from build123d import *

# Parameters (mm, degrees)
SKETCH_1_W      = 11.1
SKETCH_1_H      = 9.9
EXTRUDE_1_DEPTH = 5
SKETCH_1_3_W    = 7
SKETCH_1_3_H    = 9.9
EXTRUDE_2_DEPTH = 10
CHAMFER_1_SIZE  = 1


with BuildPart() as part:
    # 스케치1 → 보스-돌출1 (new body)
    with BuildSketch(Plane.XY):
        Rectangle(SKETCH_1_W, SKETCH_1_H)
    extrude(amount=EXTRUDE_1_DEPTH)

    # 스케치1<3> → 보스-돌출2 (add)
    with BuildSketch(Plane.XY):
        with Locations((-9.05, 0)):
            Rectangle(SKETCH_1_3_W, SKETCH_1_3_H)
        with Locations((9.05, 0)):
            Rectangle(SKETCH_1_3_W, SKETCH_1_3_H)
    extrude(amount=EXTRUDE_2_DEPTH)

    # 모따기1
    chamfer_1_edges = [part.edges().sort_by_distance(p)[0] for p in [
        (-12.55, 0, 0),
        (12.55, 0, 0),
    ]]
    chamfer(chamfer_1_edges, length=CHAMFER_1_SIZE)


solid = part.part
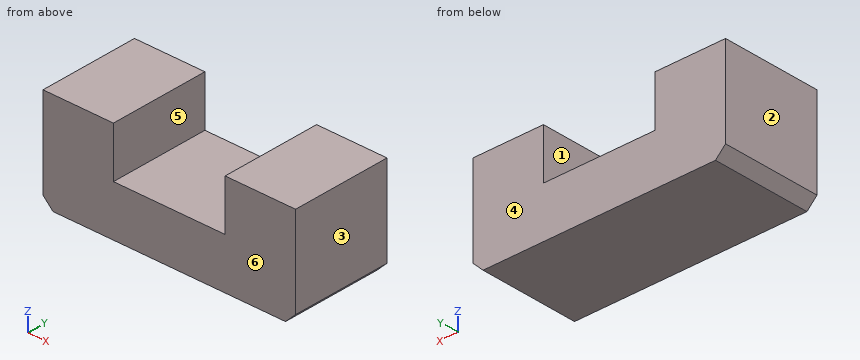
The listing builds one solid part. Answer for the finished solid, in the listing's coordinates (mm). Face numbers are marked on the shaded views. A direction names the side the tool comes from. Round coordinates to 2 decimals unless told otherwise and drop trailing zeros. Write each loop counter-clockwise with the first axis right and the second up, starting at its lowest first coordinate (ties: lowest second). Pieces come first, ordered by that corner, then holes. Notation, with made-up numbers: M 38.25,-16 L 72.25,-16 A11 ccw 72.25,4 Z; hole C 24,39 d8. An arc over 180 degrees is marked long. Write each question's results on one line, items separated by ' | '. Start each with the question number.
(1) Determine the mould class of the marked faces 1, 2, 3 and 4 for opening direction X: +X half, -X half, draft (parallel to the pull), parting line (faces both ways), or undercut.
(2) The part is cut by section B-B, the plane y = -2. Write down the section's boundary in (x, z).
(3) For the marked faces 5 and 6, determine the directions among +Z, -Z, +X, -X, +Y, -Y from which every point of the face is accessible in a straight line to the end or side of a thin tool.
(4) The part is cut by section A-A, the plane z = 6.5. Write down the section's boundary in (x, y), and give its area (3 significant figures).
(5) The part is cut by section C-C, the plane x = -1.75. Write down the section's boundary in (y, z), and give its area (3 significant figures).
(6) Find the intervals of material crossed by line 1 (X direction, y = 2, z = 6); line 2 (Z direction, x = 0.5, y = -1), in increasing order.
Worked answers:
1) face 1: undercut | face 2: -X half | face 3: +X half | face 4: draft
2) outline: M -12.55,1 L -11.55,0 L 11.55,0 L 12.55,1 L 12.55,10 L 5.55,10 L 5.55,5 L -5.55,5 L -5.55,10 L -12.55,10 Z
3) face 5: +Z, +Y, -Y | face 6: +Z, -Z, +X, -X, -Y
4) outline: M -12.55,-4.95 L -5.55,-4.95 L -5.55,4.95 L -12.55,4.95 Z; M 5.55,-4.95 L 12.55,-4.95 L 12.55,4.95 L 5.55,4.95 Z | area: 139 mm²
5) outline: M -4.95,0 L 4.95,0 L 4.95,5 L -4.95,5 Z | area: 49.5 mm²
6) line 1: x = -12.55 to -5.55, 5.55 to 12.55 | line 2: z = 0 to 5
